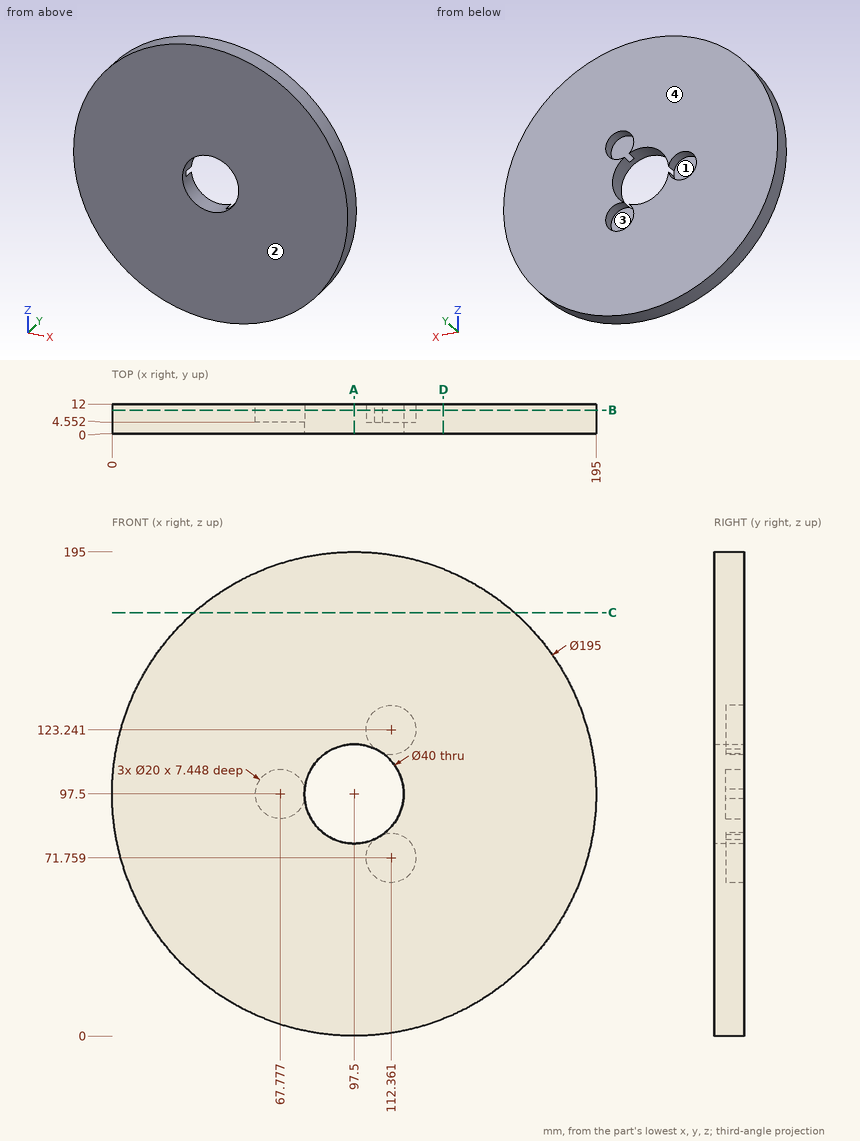
Answer from the drawing. Dimensions are ordinates in mm from the lowest x, y and z of the part. A direction names the side the tool comes from. Give positions to 0.01 mm unless a question says otherwise; leave off trailing zeros. Loops run counter-clockwise (first coordinate to the right, second up) from the corner with the lowest first, then second, coordinate; pieces in that order, holes last. Notation, with made-up numbers: (-33.75, 2) -> (11.25, 2) arc R24 ccw to (11.25, 33) -> close; hole circle Ø9 at (1, 10). An arc over 180 degrees is marked (long way). One line per question, with ' | ' between items. Start each with the question number.
1) Section C-C, the plane z = 170.5 is taken. Determine the outline of the cut face in (x, y).
2) Straight lines are drawn through the part: L1, parallel to Z at x = 103.5, y = 9.25 (1 decimal); L2, parallel to X at y = 3.5, z = 97.5; L3, parallel to X at y = 10, z = 97.5. For each, find the intervals that lie inside material, in ascending order.
3) Section D-D, the plane x = 133.5 is taken. Determine the outline of the cut face in (y, z).
4) For the marked faces 1 and 2, determine the directions among +Z, -Z, +X, -X, +Y, -Y from which every point of the face is accessible in a straight line to the end or side of a thin tool.
5) Section B-B, the plane y = 9.5 is taken. Determine the outline of the cut face in (x, z) (1 decimal).
6) Each of these flat-tipped pins is pushed along its axis until it touches: pin 1 (6 mm diameter, centred on x = 66.5, z = 97, fed in from -Y); pin 2 (4 mm diameter, centred on y = 10.5, z = 71.5, fed in from -X); pin 3 (10 mm diameter, centred on x = 69.5, z = 100.5, fed in from +Y); pin 4 (6 mm diameter, centred on x = 91.5, y = 3, fed in from -Z). Where does it stop, or does it pass through?
7) Section A-A, the plane x = 97.5 is taken. Determine the outline of the cut face in (y, z).
8) Determine the mould class of the marked faces 3 and 4 for opening direction Z: +Z half, -Z half, draft (parallel to the pull), parting line (faces both ways), or undercut.
Resolved:
1) outline: (32.87, 0) -> (162.13, 0) -> (162.13, 12) -> (32.87, 12) -> close
2) L1: 0.2 to 67.1, 76.4 to 78.4, 116.6 to 118.6, 127.9 to 194.8 | L2: 0 to 77.5, 117.5 to 195 | L3: 0 to 57.78, 117.5 to 195
3) outline: (0, 6.89) -> (12, 6.89) -> (12, 188.11) -> (0, 188.11) -> close
4) face 1: +Y | face 2: +Z, -Z, +X, -X, -Y
5) outline: circle Ø195 at (97.5, 97.5); hole (77.6, 95.6) arc R20 ccw to (105.8, 79.3) arc R10 ccw (long way) to (109.1, 81.2) arc R20 ccw to (109.1, 113.8) arc R10 ccw (long way) to (105.8, 115.7) arc R20 ccw to (77.6, 99.4) arc R10 ccw (long way) to start
6) pin 1: y = 0 | pin 2: x = 3 | pin 3: y = 4.55 | pin 4: z = 0.05
7) outline: (0, 0) -> (12, 0) -> (12, 77.5) -> (0, 77.5) -> close; (0, 117.5) -> (12, 117.5) -> (12, 195) -> (0, 195) -> close
8) face 3: undercut | face 4: draft
